```python
from build123d import *

# Parameters (mm, degrees)
SKETCH1_W                                           = 279
SKETCH1_H                                           = 85
BOSS_EXTRUDE1_DEPTH                                 = 5
CBORE_FOR_4_BINDING_HEAD_MACHINE_SCREW1_D           = 3.4544
CBORE_FOR_4_BINDING_HEAD_MACHINE_SCREW1_CBORE_D     = 6.74624
CBORE_FOR_4_BINDING_HEAD_MACHINE_SCREW1_CBORE_DEPTH = 1.7272
F_4_40_TAPPED_HOLE1_D                               = 2.2606
F_4_40_TAPPED_HOLE1_DEPTH                           = 7.6
F_4_40_TAPPED_HOLE1_TIP                             = 0.679152758
F_4_40_TAPPED_HOLE2_D                               = 2.2606
F_4_40_TAPPED_HOLE2_DEPTH                           = 7.6
F_4_40_TAPPED_HOLE2_TIP                             = 0.679152758
F_4_40_TAPPED_HOLE3_D                               = 2.2606
F_4_40_TAPPED_HOLE3_DEPTH                           = 7.6
F_4_40_TAPPED_HOLE3_TIP                             = 0.679152758


with BuildPart() as part:
    # Sketch1 → Boss-Extrude1 (new body)
    with BuildSketch(Plane.XY):
        with Locations((8.503783102, 35.532786885)):
            Rectangle(SKETCH1_W, SKETCH1_H)
    extrude(amount=BOSS_EXTRUDE1_DEPTH)

    # CBORE for #4 Binding Head Machine Screw1 (through all)
    with Locations(Plane.XY.offset(5)):
        with Locations((-116.496216898, -1.967213115), (8.503783102, -1.967213115), (133.503783102, -1.967213115)):
            CounterBoreHole(CBORE_FOR_4_BINDING_HEAD_MACHINE_SCREW1_D / 2, CBORE_FOR_4_BINDING_HEAD_MACHINE_SCREW1_CBORE_D / 2, CBORE_FOR_4_BINDING_HEAD_MACHINE_SCREW1_CBORE_DEPTH)

    # #4-40 Tapped Hole1
    with Locations(Plane.ZY.offset(130.996216898)):
        with Locations((2.5, 63.032786885), (2.5, 35.532786885), (2.5, 8.032786885)):
            Hole(F_4_40_TAPPED_HOLE1_D / 2, depth=F_4_40_TAPPED_HOLE1_DEPTH)
            with Locations((0, 0, -(F_4_40_TAPPED_HOLE1_DEPTH + F_4_40_TAPPED_HOLE1_TIP / 2))):  # 118° drill point
                Cone(0, F_4_40_TAPPED_HOLE1_D / 2, F_4_40_TAPPED_HOLE1_TIP, mode=Mode.SUBTRACT)

    # #4-40 Tapped Hole2
    with Locations(Plane(origin=(148.003783102, 0, 0), x_dir=(0, 0, -1), z_dir=(1, 0, 0))):
        with Locations((-2.5, 63.032786885), (-2.5, 35.532786885), (-2.5, 8.032786885)):
            Hole(F_4_40_TAPPED_HOLE2_D / 2, depth=F_4_40_TAPPED_HOLE2_DEPTH)
            with Locations((0, 0, -(F_4_40_TAPPED_HOLE2_DEPTH + F_4_40_TAPPED_HOLE2_TIP / 2))):  # 118° drill point
                Cone(0, F_4_40_TAPPED_HOLE2_D / 2, F_4_40_TAPPED_HOLE2_TIP, mode=Mode.SUBTRACT)

    # #4-40 Tapped Hole3
    with Locations(Plane(origin=(0, 78.032786885, 0), x_dir=(1, 0, 0), z_dir=(0, 1, 0))):
        with Locations((-91.496216898, -2.5), (108.503783102, -2.5)):
            Hole(F_4_40_TAPPED_HOLE3_D / 2, depth=F_4_40_TAPPED_HOLE3_DEPTH)
            with Locations((0, 0, -(F_4_40_TAPPED_HOLE3_DEPTH + F_4_40_TAPPED_HOLE3_TIP / 2))):  # 118° drill point
                Cone(0, F_4_40_TAPPED_HOLE3_D / 2, F_4_40_TAPPED_HOLE3_TIP, mode=Mode.SUBTRACT)


solid = part.part
```
CAD build for the part. Positions are in the model's coordinates, mm. A direction names the side the tool comes from. Coordinates: 2 decimals unless noted, no trailing zeros. Return JSON: item names as keys, results as strings. Group by question number.
Q1. Drill centre lines: line 1 (Y direction, x = -127.5, z = 2.5); line 2 (X direction, y = -3, z = 2.3); line 3 (X direction, y = 9, z = 2.55). Where is each one in solid material? Low to high.
Q2. Flat gauge pins, fed straight in: pin 1 (1.8 mm diameter, centred on y = 8.03, z = 2.5, fed in from +X); pin 2 (3 mm diameter, centred on y = 63.03, z = 2.5, fed in from +X); pin 3 (3.5 mm diameter, centred on x = -115.5, y = -2.5, fed in from +Z); pin 4 (1.4 mm diameter, centred on x = 108.5, z = 2.5, fed in from +Y). Where does each tip first touch, or does it go through?
Q3. Pull direction Y, two halves, no side cores. Call faces 3 (the face through (148.004, 35, 1)), 4 (the face through (-117, 0, 3.273)), 5 (the face through (7, -6.967, 2)): released by +Y, released by -Y, zero draft, split by the parting line, or undercut.
Q4. Which spindle directions (+Z, -Z, +X, -X, +Y, -Y) get a long thin tool onto all of the face, cutting with end or side? Do faces 1 (the face through (7, 36, 5)), 2 (the face through (133, 0, 3.273)). Say none if no direction does.
Returned:
{
 "1": {"line 1": "y = -6.97 to 6.9, 9.16 to 34.4, 36.66 to 61.9, 64.16 to 78.03", "line 2": "x = -131 to -117.88, -115.11 to 7.12, 9.89 to 132.12, 134.89 to 148", "line 3": "x = -123.3 to 140.31"},
 "2": {"pin 1": "stops at x = 140.27", "pin 2": "stops at x = 148", "pin 3": "stops at z = 3.27", "pin 4": "stops at y = 70.18"},
 "3": {"face 3": "zero draft", "face 4": "undercut", "face 5": "released by -Y"},
 "4": {"face 1": "+Z, +X, -X, +Y, -Y", "face 2": "+Z"}
}
